```python
from build123d import *
from build123d.topology import SkipClean

# Parameters (mm, degrees)
CORTAR_EXTRUIR7_REACH      = 34.904
CORTAR_EXTRUIR7_END_RADIUS = 4.5
CROQUIS17_R                = 1.5
CORTAR_EXTRUIR10_START     = -3
CORTAR_EXTRUIR10_DEPTH     = 6
CROQUIS21_W                = 3.1
CROQUIS21_H                = 3.480038904
CHAFL_N2_SIZE              = 0.5
CROQUIS22_W                = 60
CROQUIS22_H                = 60
SALIENTE_EXTRUIR1_DEPTH    = 3
REDONDEO1_R                = 2
CROQUIS23_R                = 1.5
CROQUIS23_W                = 15
CROQUIS23_H                = 45
CORTAR_EXTRUIR11_DEPTH     = 2


with BuildPart() as part:
    # Croquis9 → Revolución3 (revolve)
    with BuildSketch(Plane.XY, mode=Mode.PRIVATE) as revoluci_n3_sk:
        Polygon((0, 10.708007251), (-22, 10.708007251), (-22, 7.708007251), (-13.488403702, 7.708007251), (-4.5, 6.708007251), (-4.5, -1.291992749), (0, -1.291992749), align=None)
    revolve(revoluci_n3_sk.sketch.rotate(Axis((0, 17.712309747, 0), (0, -1, 0)), 270), axis=Axis((0, 17.712309747, 0), (0, -1, 0)))

    # Cortar-Extruir7: up to this cylinder (the profile starts inside it)
    cortar_extruir7_end = Plane(origin=(0, 4.708007, 0), z_dir=(0, 1, 0)) * Cylinder(CORTAR_EXTRUIR7_END_RADIUS, 79.808, mode=Mode.PRIVATE)
    # Croquis17 → Cortar-Extruir7 (cut, up to the surface)
    with BuildSketch(Plane(origin=(0, 0, 0), x_dir=(0, 0, -1), z_dir=(1, 0, 0)), mode=Mode.PRIVATE) as cortar_extruir7_sk1:
        with Locations(Location((0, 4.708007251, 0), (0, 0, 180))):
            Circle(CROQUIS17_R)
    cortar_extruir7_tool1 = extrude(cortar_extruir7_sk1.sketch, amount=CORTAR_EXTRUIR7_REACH, mode=Mode.PRIVATE) & cortar_extruir7_end
    add(cortar_extruir7_tool1.solids().sort_by_distance((0, 4.708007, 0))[0], mode=Mode.SUBTRACT)

    # Croquis18 → Cortar-Extruir10 (cut)
    with BuildSketch(Plane(origin=(0, 10.708007251, 0), x_dir=(1, 0, 0), z_dir=(0, 1, 0)).offset(CORTAR_EXTRUIR10_START)):
        with BuildLine():
            Line((1, 2.93428015), (1, -2.93428015))
            ThreePointArc((1, -2.93428015), (-3.1, 0), (1, 2.93428015))
        make_face()
    extrude(amount=-CORTAR_EXTRUIR10_DEPTH, mode=Mode.SUBTRACT)

    # Croquis21 → Cortar-Revolución1 (revolve, cut)
    with SkipClean():  # the faces are left unmerged after this step: merging them gives an invalid solid
        with BuildSketch(Plane.XY, mode=Mode.PRIVATE) as cortar_revoluci_n1_sk:
            with Locations((-1.55, 0.068456853)):
                Rectangle(CROQUIS21_W, CROQUIS21_H)
        revolve(cortar_revoluci_n1_sk.sketch.rotate(Axis((0, 3.581140077, 0), (0, -1, 0)), 251.180936631), axis=Axis((0, 3.581140077, 0), (0, -1, 0)), mode=Mode.SUBTRACT)

    # Chaflán2
    # the kernel refuses this chamfer: 0.5 mm, written as the material it takes off along each edge
    with BuildSketch(Plane(origin=(1, 1.808476305, 4.220121644), x_dir=(-0.02749587661058627, 0.9996219169112968, 0), z_dir=(0, 0, -1))) as chafl_n2_piece_1_section:
        Polygon((CHAFL_N2_SIZE * 0.999621916911, CHAFL_N2_SIZE * 0.0274958766106), (-CHAFL_N2_SIZE * 0.0274958766106, CHAFL_N2_SIZE * 0.999621916911), (0, 0), align=None)
    chafl_n2_piece_1 = extrude(amount=8.440243288, mode=Mode.PRIVATE)
    chafl_n2_piece_1 = chafl_n2_piece_1 & Plane(origin=(0, 1.974615601, 0), x_dir=(0.32258064516148965, 0, 0.946541983943236), z_dir=(0, -1, 0)) * Cylinder(3.1, 19, mode=Mode.PRIVATE)
    add(chafl_n2_piece_1, mode=Mode.SUBTRACT)

    # Croquis22 → Saliente-Extruir1 (add)
    with BuildSketch(Plane(origin=(0, 10.708007251, 0), x_dir=(1, 0, 0), z_dir=(0, 1, 0))):
        Rectangle(CROQUIS22_W, CROQUIS22_H)
    extrude(amount=-SALIENTE_EXTRUIR1_DEPTH)

    # Redondeo1
    redondeo1_edges = [part.edges().sort_by_distance(p)[0] for p in [
        (-30, 9.208007251, -30),
        (-30, 9.208007251, 30),
        (30, 9.208007251, 30),
        (30, 9.208007251, -30),
    ]]
    fillet(redondeo1_edges, radius=REDONDEO1_R)

    # Croquis23 → Cortar-Extruir11 (cut)
    with BuildSketch(Plane(origin=(0, 10.708007251, 0), x_dir=(1, 0, 0), z_dir=(0, 1, 0))):
        with Locations(Location((-26, 24, 0), (0, 0, 270))):
            Circle(CROQUIS23_R)
        with Locations(Location((-26, -24, 0), (0, 0, 270))):
            Circle(CROQUIS23_R)
        with Locations(Location((26, -24, 0), (0, 0, 270))):
            Circle(CROQUIS23_R)
        with Locations(Location((26, 24, 0), (0, 0, 270))):
            Circle(CROQUIS23_R)
        with Locations((2.713645645, -2.5)):
            Rectangle(CROQUIS23_W, CROQUIS23_H)
    extrude(amount=-CORTAR_EXTRUIR11_DEPTH, mode=Mode.SUBTRACT)


solid = part.part
```
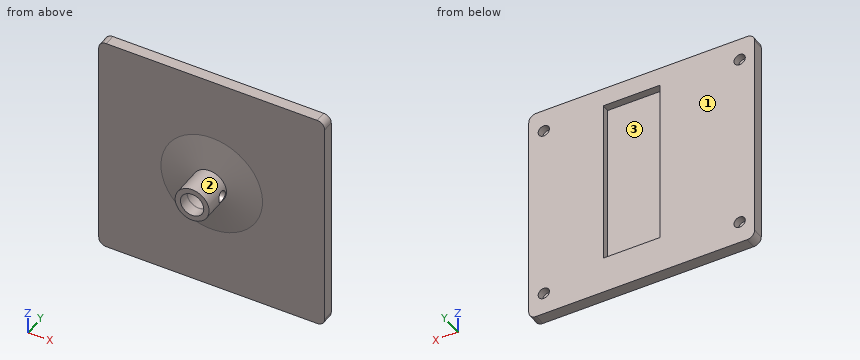
Work out the finished part from the listing and answer in its coordinate system (mm). Face numbers are marked on the shaded views. Coordinates: 2 decimals unless noted, no trailing zeros. Order: outer loops, then holes, each group sorted by start corner. A loop starts at its lowest first (then second) coordinate and runs counter-clockwise, first axis right, second up. Notation, with made-up numbers: M 74,52 L 88,52 A28 cw 88,76 Z; hole C 37,9.25 d10. An arc over 180 degrees is marked long. Use CSV: the item, a comma, the result in double quotes.
1) Flat-ended cylindrical pins translate along their axes: pin 1 Ø1 at (y, z) = (1, 2) entering from +X; pin 2 Ø1.8 at (y, z) = (4.71, 0) entering from +X; pin 3 Ø2.5 at (x, z) = (26, 24) entering from +Y. Find the tip coordinate at first contact, or state that the pin passes through.
Worked out:
pin 1,"stops at x = 4.24"
pin 2,"stops at x = -2.97"
pin 3,"stops at y = 8.71"
2) Section A-A on z = 0 is taken. Write down the section's boundary in (x, y), plus the area to 3 significant figures.
Worked out:
outline,"M -30,7.71 L -13.49,7.71 L -4.5,6.71 L -4.5,-1.29 L -3.1,-1.29 L -3.1,7.71 L 1,7.71 L 1,6.21 L 4.5,6.21 L 4.5,6.71 L 13.49,7.71 L 30,7.71 L 30,10.71 L 10.21,10.71 L 10.21,8.71 L -4.79,8.71 L -4.79,10.71 L -30,10.71 Z; M 1,2.31 L 1.5,1.81 L 3.1,1.81 L 3.1,-1.29 L 4.5,-1.29 L 4.5,3.21 L 1,3.21 Z"
area,"186 mm^2"
3) Section D-D on z = -15 is taken. Write down the section's boundary in (x, y).
Worked out:
outline,"M -30,7.71 L 30,7.71 L 30,10.71 L 10.21,10.71 L 10.21,8.71 L -4.79,8.71 L -4.79,10.71 L -30,10.71 Z"
4) Section B-B on y = 9.5 is taken. Write down the section's boundary in (x, z), plus the area to 3 significant figures.
Worked out:
outline,"M -30,-28 A2 ccw -28,-30 L 28,-30 A2 ccw 30,-28 L 30,28 A2 ccw 28,30 L -28,30 A2 ccw -30,28 Z; hole C -26,-24 d3; hole C -26,24 d3; hole M -4.79,-20 L 10.21,-20 L 10.21,25 L -4.79,25 Z; hole C 26,-24 d3; hole C 26,24 d3"
area,"2,890 mm^2"
5) Section C-C on x = 0 is taken. Write down the section's boundary in (y, z).
Worked out:
outline,"M -1.29,-4.5 L 6.71,-4.5 L 7.71,-13.49 L 7.71,-30 L 10.71,-30 L 10.71,-20 L 8.71,-20 L 8.71,25 L 10.71,25 L 10.71,30 L 7.71,30 L 7.71,13.49 L 6.71,4.5 L -1.29,4.5 L -1.29,3.1 L 7.71,3.1 L 7.71,-3.1 L -1.29,-3.1 Z"
6) Determine the mould class of the marked faces 1, 2 and 3 for opening direction X: released by +X, released by -X, zero draft, split by the parting line, or undercut.
Worked out:
face 1,"zero draft"
face 2,"split by the parting line"
face 3,"undercut"
7) Consider line 1 (Z direction, x = 6, y = 10); line 2 (X direction, y = 6.5, z = 0); line 3 (X direction, y = 9.8, z = 24). Determine where each line is inside the solid, lowest interval first. Write a range as [from, to].
Worked out:
line 1,"z = [-30, -20], [25, 30]"
line 2,"x = [-4.5, -3.1], [1, 4.5]"
line 3,"x = [-30, -27.5], [-24.5, -4.79], [10.21, 24.5], [27.5, 30]"
